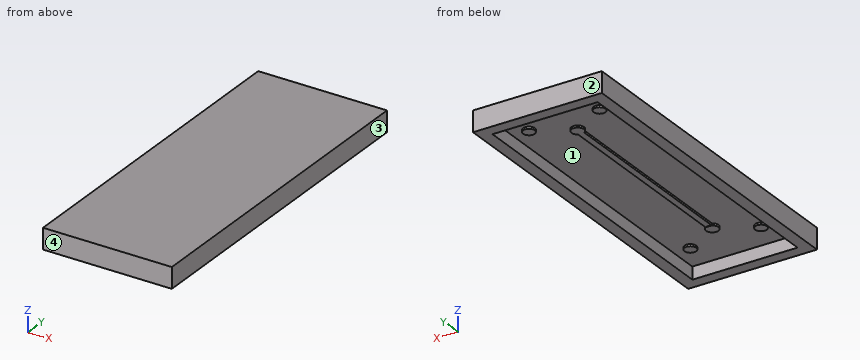
Autodesk Inventor part; units mm, degrees
ref_plane "Arbeitsebene2" through (-2, 9.25, -0.4) normal (0, 0, 1) x (1, 0, 0)
ref_plane "YZ Plane" through (0, 0, 0) normal (1, 0, 0) x (0, 1, 0)
ref_plane "XZ Plane" through (0, 0, 0) normal (0, 1, 0) x (-1, 0, 0)
ref_plane "Arbeitsebene1" through (0, 0, 0) normal (0, 0, 1) x (1, 0, 0)
sketch "Skizze1" plane through (0, 0, 0) normal (0, 0, 1) x (1, 0, 0)
  line L0 (12.5, -37) -> (-12.5, -37)
  line L1 (12.5, 37) -> (12.5, -37)
  line L2 (-12.5, 37) -> (12.5, 37)
  line L3 (-12.5, -37) -> (-12.5, 37)
  circle A0 centre (-8.5, -30) radius 1.4
  circle A1 centre (8.5, -30) radius 1.4
  circle A2 centre (8.5, 30) radius 1.4
  circle A3 centre (-8.5, 30) radius 1.4
  line L4 (-0.75, 23.146) -> (-0.75, -23.146)
  arc A4 (0.75, 23.146) -> (-0.75, 23.146) centre (0, 25) ccw
  line L5 (0.75, -23.146) -> (0.75, 23.146)
  arc A5 (-0.75, -23.146) -> (0.75, -23.146) centre (0, -25) ccw
  line L6 (15.5, -40) -> (-15.5, -40)
  line L7 (-15.5, -40) -> (-15.5, 40)
  line L8 (-15.5, 40) -> (15.5, 40)
  line L9 (15.5, 40) -> (15.5, -40)
  point P0 (0, 0)
  dimension "d0" = 3
extrude "Extrusion1" add sketch "Skizze1" along normal blind 2 contours L0 L3 L2 L1 | A0 | A1 | A2 | A3 | A4 L5 A5 L4 | L6 L7 L8 L9
ref_plane "Arbeitsebene2" through (-2, 9.25, -0.4) normal (0, 0, 1) x (1, 0, 0)
sketch "Skizze2" plane through (0, 0, 0) normal (0, 0, -1) x (-1, 0, 0)
  circle A0 centre (0, -25) radius 2.5 construction
  circle A1 centre (0, 25) radius 2.5 construction
  line L0 (12.5, -37) -> (12.5, 37)
  line L1 (12.5, 37) -> (-12.5, 37)
  line L2 (-12.5, 37) -> (-12.5, -37)
  line L3 (-12.5, -37) -> (12.5, -37)
  circle A2 centre (8.5, -30) radius 1.4
  circle A3 centre (-8.5, -30) radius 1.4
  circle A4 centre (-8.5, 30) radius 1.4
  circle A5 centre (8.5, 30) radius 1.4
  line L4 (0.75, -7.25) -> (0.75, -23.146) construction
  line L5 (-0.75, 7.25) -> (-0.75, 23.146) construction
  line L6 (0.75, -7.25) -> (0.75, -23.146) construction
  line L7 (-0.75, 7.25) -> (-0.75, 23.146) construction
  circle A6 centre (0, -25) radius 2.5 construction
  circle A7 centre (0, 25) radius 2.5 construction
  circle A8 centre (0, 25) radius 32.2587 construction
  circle A9 centre (0, -25) radius 2 construction
  circle A10 centre (0, 25) radius 1.5
  circle A11 centre (0, -25) radius 1.5
  line L8 (0.75, 23.701) -> (-0.75, 23.701)
  line L9 (-0.75, 23.701) -> (-0.75, -23.701)
  line L10 (-0.75, -23.701) -> (0.75, -23.701)
  line L11 (0.75, -23.701) -> (0.75, 23.701)
  line L12 (-9.25, 9.25) -> (9.25, 9.25)
  line L13 (9.25, 9.25) -> (9.25, -9.25)
  line L14 (9.25, -9.25) -> (-9.25, -9.25)
  line L15 (-9.25, -9.25) -> (-9.25, 9.25)
  point P0 (0, 0)
  point P1 (-0.75, 22.6152)
  point P2 (-0.75, -22.6152)
  point P3 (0.75, -22.6152)
  point P4 (0.75, 22.6152)
  point P5 (-0.75, -23.146)
extrude "Extrusion2" add sketch "Skizze2" along normal blind 0.5 contours A2 | A3 | A4 | A5 | A10 L8 | L8 A10 | A10 L11 L12 L9 | L12 L11 L14 L9 | L14 L11 A11 L9 | L10 A11 picked at (0.3855, -25.1784)
sketch "Skizze4" plane through (0, 0, 0) normal (0, 0, -1) x (-1, 0, 0)
  circle A0 centre (8.5, -30) radius 1.4
  circle A1 centre (-8.5, 30) radius 1.4
  arc A2 (0.75, 23.701) -> (-0.75, 23.701) centre (0, 25) ccw
  line L0 (0.75, 23.701) -> (0.75, -23.701)
  arc A3 (-0.75, -23.701) -> (0.75, -23.701) centre (0, -25) ccw
  line L1 (-0.75, -23.701) -> (-0.75, 23.701)
  circle A4 centre (-8.5, -30) radius 1.4
  circle A5 centre (8.5, 30) radius 1.4
  line L2 (-15.5, 40) -> (15.5, 40)
  line L3 (-15.5, -40) -> (-15.5, 40)
  line L4 (15.5, -40) -> (-15.5, -40)
  line L5 (15.5, 40) -> (15.5, -40)
  line L6 (12.65, 37.15) -> (-12.65, 37.15)
  line L7 (-12.65, 37.15) -> (-12.65, -37.15)
  line L8 (-12.65, -37.15) -> (12.65, -37.15)
  line L9 (12.65, -37.15) -> (12.65, 37.15)
  point P0 (0, 0)
  dimension "d11" = 2.85
extrude "Extrusion4" add sketch "Skizze4" along normal blind 3 contours L2 L5 L4 L3
properties part number "40_microfluidic_chip_lightsheet_layer1_negative_mould_upper_v0"
Verification items for the finished model (mm, model axes). Face numbers are marked on the shaded views. Coordinates: 2 decimals unless noted, no trailing zeros. Loops run counter-clockwise (first coordinate to the right, second up) from the corner with the lowest first, then second, coordinate; pieces in that order, holes last. Notation, with made-up numbers: (31.5, 84.5) - (87.5, 84.5) arc R20 cw to (87.5, 97.5) - close; hole circle Ø8 at (-10.75, 41.25). An arc over 180 degrees is marked (long way). Return JSON: item names as keys, results as strings.
1. Mould release check, pull along Y, two halves, no side actions. Record for the marked faces 1, 2, 3 and 4: +Y half, -Y half, draft (parallel to the pull), parting line (faces both ways), or undercut.
Established:
{"face 1": "undercut", "face 2": "+Y half", "face 3": "draft", "face 4": "-Y half"}
2. Go/stop test with flat-tipped pins: pin 1 (0.8 mm diameter, centred on x = 8, y = -30, fed in from -Z); pin 2 (5 mm diameter, centred on x = -8.5, y = 8.5, fed in from -Z). Record where each tip stops, or that it passes through.
Established:
{"pin 1": "stops at z = -0.5", "pin 2": "stops at z = 0"}
3. Section check C-C, the plane y = -25. Record the boundary of the cut face in (x, z), then the cut area to 3 significant figures.
Established:
{"outline": "(-15.5, -3) - (-12.65, -3) - (-12.65, 0) - (-1.5, 0) - (-1.5, -0.5) - (1.5, -0.5) - (1.5, 0) - (12.65, 0) - (12.65, -3) - (15.5, -3) - (15.5, 2) - (-15.5, 2) - close", "area": "80.6 mm2"}
4. Section check A-A, the plane z = -1.35. Record the boundary of the cut face in (x, y), then the cut area to 3 significant figures.
Established:
{"outline": "(-15.5, -40) - (15.5, -40) - (15.5, 40) - (-15.5, 40) - close; hole (-12.65, -37.15) - (12.65, -37.15) - (12.65, 37.15) - (-12.65, 37.15) - close", "area": "600 mm2"}
5. Section check B-B, the plane x = 0. Record the boundary of the cut face in (y, z).
Established:
{"outline": "(-40, -3) - (-37.15, -3) - (-37.15, 0) - (-26.5, 0) - (-26.5, -0.5) - (-23.7, -0.5) - (-23.7, 0) - (-23.5, 0) - (-23.5, -0.5) - (26.5, -0.5) - (26.5, 0) - (37.15, 0) - (37.15, -3) - (40, -3) - (40, 2) - (-40, 2) - close"}
6. Thickness scan on L1, parallel to Y at x = 2, z = -1.2; L2, parallel to X at y = -2, z = -1; L3, parallel to Z at x = -6, y = 8. Record the ranges inside material, lowest first.
Established:
{"L1": "y = -40 to -37.15, 37.15 to 40", "L2": "x = -15.5 to -12.65, 12.65 to 15.5", "L3": "z = 0 to 2"}
7. Section check D-D, the plane x = 8.5. Record the boundary of the cut face in (y, z), then the cut area to 3 significant figures.
Established:
{"outline": "(-40, -3) - (-37.15, -3) - (-37.15, 0) - (-31.4, 0) - (-31.4, -0.5) - (-28.6, -0.5) - (-28.6, 0) - (28.6, 0) - (28.6, -0.5) - (31.4, -0.5) - (31.4, 0) - (37.15, 0) - (37.15, -3) - (40, -3) - (40, 2) - (-40, 2) - close", "area": "180 mm2"}
